The model under review builds one solid part; all positions refer to its coordinate system, in mm. Face numbers are marked on the shaded views. Coordinates: 2 decimals unless noted, no trailing zeros. Loops run counter-clockwise (first coordinate to the right, second up) from the corner with the lowest first, then second, coordinate; pieces in that order, holes last. Notation, with made-up numbers: M 38,-11 L 75,-11 A25 cw 75,20 Z; hole C -15,22.25 d5. An arc over 180 degrees is marked long. Use CSV: the item, a comma, the result in double quotes. Start each with the question number.
1. Add section A-A, the plane z = -2.25. Write out the cut boundary in (x, y), then the cut area to 3 significant figures.
2. Draft analysis for pull direction Y (two halves, no side actions). For the marked faces 1 and 2, state which applies: +Y half, -Y half, draft (parallel to the pull), parting line (faces both ways), or undercut.
3. Clearance check with flat-ended pins moving along their axes: P1, Ø1.5, axis at y = -8, z = 2.5, coming from the +X side; P2, Ø4, axis at x = -5.5, z = -1, coming from the +Y side; P3, Ø3, axis at y = 6, z = 2.5, coming from the -X side; P4, Ø10, axis at x = -7.5, y = 3, coming from the -Z side. State where each tip first meets the part, or that it passes through.
4. For L1, parallel to Y at x = -10.25, z = 0.5; L2, parallel to Y at x = -10.2, z = -0.25; L3, parallel to X at y = 1.5, z = 1, list the stretches that pass through material, from the lowest coordinate up.
from build123d import *

# Parameters (mm, degrees)
F3_R     = 11.75
F5_DEPTH = 0.75
F2_R     = 18.1470501703
F7_ANGLE = 5


with BuildPart() as f1:
    # F0 (on Front) → F1 (revolve)
    with BuildSketch(Plane.XZ):
        with BuildLine():
            Line((0, 3.25), (0, 0))
            Line((0, 0), (0, -3.25))
            ThreePointArc((0, -3.25), (0.0732233047, -3.4267766953), (0.25, -3.5))
            Line((0.25, -3.5), (0.6801960973, -3.5))
            ThreePointArc((0.6801960973, -3.5), (1.3141850029, -3.2733421413), (1.660776773, -2.6961161351))
            Line((1.660776773, -2.6961161351), (1.9509344755, -1.2453276227))
            ThreePointArc((1.9509344755, -1.2453276227), (1.9654871264, -1.1477491056), (1.9703537998, -1.0492114876))
            Line((1.9703537998, -1.0492114876), (1.9703537998, 0))
            Line((1.9703537998, 0), (1.9703537998, 1.0492114876))
            ThreePointArc((1.9703537998, 1.0492114876), (1.9654871264, 1.1477491056), (1.9509344755, 1.2453276227))
            Line((1.9509344755, 1.2453276227), (1.660776773, 2.6961161351))
            ThreePointArc((1.660776773, 2.6961161351), (1.3141850029, 3.2733421413), (0.6801960973, 3.5))
            Line((0.6801960973, 3.5), (0.25, 3.5))
            ThreePointArc((0.25, 3.5), (0.0732233047, 3.4267766953), (0, 3.25))
        make_face()
    revolve(axis=Axis((-10.2, 0, 1.7540712142), (0, 0, 1)))


with BuildPart() as f5:
    # F3 (on Top) → F5 (new body)
    with BuildSketch(Plane.XY):
        with Locations((-10.2, 0)):
            Circle(F3_R)
    extrude(amount=F5_DEPTH)


with BuildPart() as f5b:
    # F2 (on Top) → F5, piece 2 (new body)
    with BuildSketch(Plane.XY):
        with Locations((-10.076363571, 0)):
            Circle(F2_R)
    extrude(amount=F5_DEPTH)

    # F6: cut F5
    add(f5.part, mode=Mode.SUBTRACT)


with BuildPart() as f5b_1:
    # F7: moved
    add(f5b.part.rotate(Axis((-10.0247794762, 17.2923859209, 0), (0, 1, 0)), F7_ANGLE))


with BuildPart() as f1_1:
    add(f1.part)

    # F8: cut F5b
    add(f5b_1.part, mode=Mode.SUBTRACT)


solid = f1_1.part
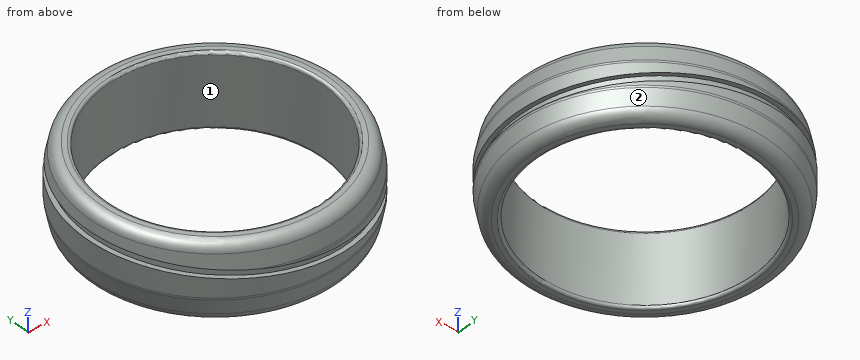
Computed:
1,outline,"C -10.2,0 d23.9; hole C -10.2,0 d20.4"
1,area,"122 mm^2"
2,face 1,"undercut"
2,face 2,"parting line"
3,P1,"stops at x = -0.73"
3,P2,"stops at y = 11.87"
3,P3,"stops at x = -21.3"
3,P4,"passes through"
4,L1,"y = -11.75 to -10.2, 10.2 to 11.75"
4,L2,"y = -12.17 to -10.2, 10.2 to 12.17"
4,L3,"x = -22.28 to -20.29, -0.11 to 1.88"
